from build123d import *

# Parameters (mm, degrees)
F1_DEPTH = 63.5
F0_W     = 22.693397
F0_H     = 19.05
F2_DEPTH = 25.4
F3_DEPTH = 7.9375
F5_R     = 6.35


with BuildPart() as f1:
    # F0 (on Front) → F1 (new body, symmetric)
    with BuildSketch(Plane.XZ):
        Polygon((41.275, -9.525), (41.275, 9.525), (22.225, 9.525), (-41.275, 9.525), (-41.275, -9.525), align=None)
    extrude(amount=F1_DEPTH, both=True)

    # F0 (on Front) → F2 (join, symmetric)
    with BuildSketch(Plane.XZ):
        with BuildLine():
            Line((22.225, 9.525), (41.275, 9.525))
            Line((41.275, 9.525), (41.275, 46.0502))
            ThreePointArc((41.275, 46.0502), (45.92468, 57.27552), (57.15, 61.9252))
            Line((57.15, 61.9252), (63.031603, 61.9252))
            Line((63.031603, 61.9252), (63.031603, 80.9752))
            Line((63.031603, 80.9752), (57.15, 80.9752))
            ThreePointArc((57.15, 80.9752), (32.454296, 70.745904), (22.225, 46.0502))
            Line((22.225, 46.0502), (22.225, 9.525))
        make_face()
        with Locations((74.378301, 71.4502)):
            Rectangle(F0_W, F0_H)
    extrude(amount=F2_DEPTH, both=True)

    # F0 (on Front) → F3 (join, symmetric)
    with BuildSketch(Plane.XZ):
        with BuildLine():
            Line((-41.275, 9.525), (22.225, 9.525))
            Line((22.225, 9.525), (22.225, 46.0502))
            ThreePointArc((22.225, 46.0502), (32.454296, 70.745904), (57.15, 80.9752))
            add(Edge.make_bspline(
                [(-41.275, 9.525), (-39.910629, 47.554985), (-5.663922, 81.163555), (57.15, 80.9752)],
                knots=[0, 0, 0, 0, 121.624881, 121.624881, 121.624881, 121.624881], degree=3))
        make_face()
    extrude(amount=F3_DEPTH, both=True)

    # F0 (on Front) → F4 (revolve)
    with BuildSketch(Plane.XZ):
        Polygon((88.431603, 71.4375), (88.431603, 57.15), (113.831603, 57.15), (113.831603, 85.725), (88.431603, 85.725), align=None)
    revolve(axis=Axis((88.431603, 0, 64.29375), (0, 0, -1)))

    # F5
    f5_edges = [f1.edges().sort_by_distance(p)[0] for p in [
        (-41.275, 63.5, 0),
        (-41.275, -63.5, 0),
        (41.275, -63.5, 0),
        (41.275, 63.5, 0),
    ]]
    fillet(f5_edges, radius=F5_R)


solid = f1.part
Source: CAD feature listing. Evaluate the final solid. Frame: model axes, mm. A direction names the side the tool comes from. Give positions to 0.01 mm unless a question says otherwise; leave off trailing zeros. Order: outer loops, then holes, each group sorted by start corner. A loop starts at its lowest first (then second) coordinate and runs counter-clockwise, first axis right, second up. Notation, with made-up numbers: (-15, 4) -> (26, 4) arc R33 ccw to (26, 35) -> close; hole circle Ø1 at (80.5, -3.75). An arc over 180 degrees is marked (long way). Write item = value, one per line.
Item 1: Section query A-A (y = -16.5). Output: boundary loops of the cut face in (x, z) (3 decimals), then the cut area to 3 significant figures.
Check result:
outline = (-41.275, -9.525) -> (41.275, -9.525) -> (41.275, 46.05) arc R15.875 cw to (57.15, 61.925) -> (69.121, 61.925) -> (69.121, 57.15) -> (107.742, 57.15) -> (107.742, 85.725) -> (69.121, 85.725) -> (69.121, 80.975) -> (57.15, 80.975) arc R34.925 ccw to (22.225, 46.05) -> (22.225, 9.525) -> (-41.275, 9.525) -> close
area = 4,360 mm²
Item 2: Mould query, pull axis X, two halves, no side actions, for faces 1 (the face through (45.8, -0.36, 57.15)), 2 (the face through (22.225, -17, 28)), 3 (the face through (1, 35, 9.525)). Classes: +X half, -X half, draft (parallel to the pull), parting line (faces both ways), or undercut.
Check result:
face_1 = undercut
face_2 = -X half
face_3 = draft
Item 3: Ray query, probe 1 along X at (y, z) = (56, 6.5) (3 decimals); probe 2 along Z at (x, y) = (-24, -11) (3 decimals); probe 3 along X at (y, z) = (21.5, 30.5) (3 decimals). Return the intervals inside material, ascending.
Check result:
probe_1 = -41.275 to 41.275
probe_2 = -9.525 to 9.525
probe_3 = 22.225 to 41.275
Item 4: Contact query for flat-ended pins moving along their axis: pin 1 (10 mm diameter, centred on x = 39.5, z = 28.5, fed in from -Y); pin 2 (10 mm diameter, centred on x = 43.5, y = -31, fed in from +Z) (3 decimals); pin 3 (19 mm diameter, centred on y = -18.5, z = 23, fed in from -X) (3 decimals). Output: stop coordinate, or through.
Check result:
pin_1 = -25.4
pin_2 = 9.525
pin_3 = 22.225
Item 5: Set-up query: faces 4 (the face through (1, -36, 9.525)), 5 (the face through (62, 0, 80.975)), 6 (the face through (22.225, 17, 28)). Return all of +Z, -Z, +X, -X, +Y, -Y with unobstructed straight access to the full face (end or side cutting, diameter ignored); none if empty.
Check result:
face_4 = +Z, -X, -Y
face_5 = +Z, -X
face_6 = +Z, -X, +Y
